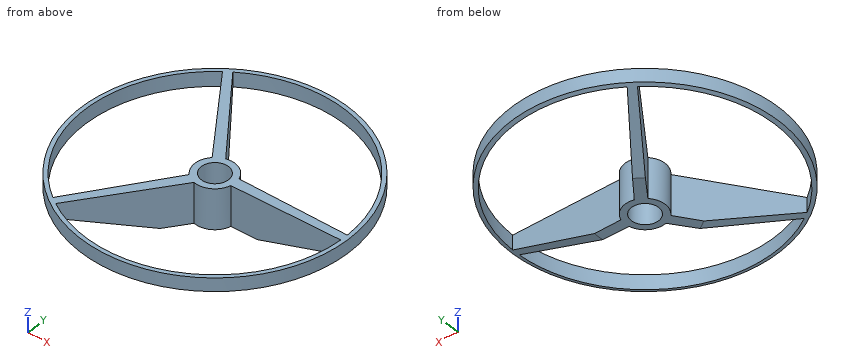
from build123d import *

# Parameters (mm, degrees)
CYLINDER_R     = 100
CYLINDER_DEPTH = 10
SKETCH_R       = 100
SKETCH_R_2     = 10.15
PAD_DEPTH      = 40


with BuildPart() as cone:
    # Cone → Cone (revolve)
    with BuildSketch(Plane(origin=(0, 0, -30), x_dir=(1, 0, 0), z_dir=(0, -1, 0))):
        Polygon((0, 0), (2, 0), (100, 30), (0, 30), align=None)
    revolve(axis=Axis((0, 0, -30), (0, 0, 1)))


with BuildPart() as fusion:
    # Cylinder → Cylinder (new body)
    with BuildSketch(Plane.XY):
        Circle(CYLINDER_R)
    extrude(amount=CYLINDER_DEPTH)

    # Fusion: union Cone
    add(cone.part)


with BuildPart() as fusion_1:
    # Fusion placement: moved
    add(fusion.part.moved(Location((0, 0, 20))))


with BuildPart() as common:
    # Sketch → Pad (new body)
    with BuildSketch(Plane.XY):
        Circle(SKETCH_R)
        Circle(SKETCH_R_2, mode=Mode.SUBTRACT)
        with BuildLine():
            ThreePointArc((96.949765, 3.121375), (44.731918, 86.070062), (-53.160067, 81.135734))
            Line((-3.811001, 14.5078), (-53.160067, 81.135734))
            ThreePointArc((14.25383, 4.672079), (7.172763, 13.173894), (-3.811001, 14.5078))
            Line((14.25383, 4.672079), (96.949765, 3.121375))
        make_face(mode=Mode.SUBTRACT)
        with BuildLine():
            Line((14.628164, -3.319158), (96.957277, -2.87862))
            ThreePointArc((-53.160067, -81.135734), (44.839635, -86.013994), (96.957277, -2.87862))
            Line((-3.811001, -14.5078), (-53.160067, -81.135734))
            ThreePointArc((-3.811001, -14.5078), (7.781336, -12.823838), (14.628164, -3.319158))
        make_face(mode=Mode.SUBTRACT)
        with BuildLine():
            Line((-10.726301, -10.485536), (-58.074672, -77.693838))
            ThreePointArc((-58.074672, 77.693838), (-97, 0), (-58.074672, -77.693838))
            Line((-10.726301, 10.485536), (-58.074672, 77.693838))
            ThreePointArc((-10.726301, 10.485536), (-15, 0), (-10.726301, -10.485536))
        make_face(mode=Mode.SUBTRACT)
    extrude(amount=PAD_DEPTH)

    # Common: intersect Fusion
    add(fusion_1.part, mode=Mode.INTERSECT)


solid = common.part
For this review, take the finished solid that the model builds, in its own axes (mm). Give positions to 0.01 mm unless a question says otherwise; leave off trailing zeros. Loops run counter-clockwise (first coordinate to the right, second up) from the corner with the lowest first, then second, coordinate; pieces in that order, holes last. Notation, with made-up numbers: M 32,-28 L 39,-28 A13 cw 39,-3 Z; hole C 61,-5 d4. An arc over 180 degrees is marked long. Answer as a JSON object with one key per item and string values. Group by question number.
Q1. Add section B-B on y = 0. Give the boundary of the cut face in (x, z).
Q2. Add section A-A on x = 0. Give the boundary of the cut face in (y, z), and give its area (3 significant figures).
Q3. For probe 1 along Y at (x, z) = (0, 18.5); probe 2 along X at (y, z) = (-71, 25.5); probe 3 along X at (y, z) = (28, 20.5), list the stretches that pass through material, from the lowest coordinate up. Write a range as [from, to].
Q4. Insertion check: P1, Ø6, axis at x = 69.5, z = 11.5, coming from the -Y side; P2, Ø5, axis at x = 56, z = 12, coming from the -Y side; P3, Ø1, axis at x = -8, z = 23.5, coming from the +Y side. Each pin has a flat end and moves straight along its axis. Give the tip position at first contact, or say it passes through.
Q5. Add section D-D on x = 85. Give the number of separate pieces and of enclosed holes in the cut face, and give its area (3 significant figures).
Q6. Add section C-C on z = 8.5. Give the boundary of the cut face in (x, y), and give its area (3 significant figures).
Checked values:
{
 "1": {"outline": "M -100,20 L -97,19.08 L -97,30 L -100,30 Z; M -15,0 L -10.15,0 L -10.15,30 L -15,30 Z; M 10.15,0 L 34.67,0 L 100,20 L 100,30 L 10.15,30 Z"},
 "2": {"outline": "M -100,20 L -97,19.08 L -97,30 L -100,30 Z; M -15,0 L -10.15,0 L -10.15,30 L -15,30 Z; M 10.15,0 L 15,0 L 15,30 L 10.15,30 Z; M 97,19.08 L 100,20 L 100,30 L 97,30 Z", "area": "354 mm²"},
 "3": {"probe 1": "[-15, -10.15], [10.15, 15]", "probe 2": "[-70.42, -66.09], [-53.36, -45.65], [66.09, 70.42]", "probe 3": "[-96, -92.87], [-23.07, -13.8], [92.87, 96]"},
 "4": {"P1": "y = -3.04", "P2": "y = -3.11", "P3": "y = 99.72"},
 "5": {"separate pieces": "3", "enclosed holes": "0", "area": "216 mm²"},
 "6": {"outline": "M -38.15,-49.42 A62.43 ccw -32.53,-53.29 L -3.81,-14.51 A15 ccw 14.63,-3.32 L 62.36,-3.06 A62.43 ccw 62.32,3.77 L 14.25,4.67 A15 ccw -3.81,14.51 L -32.53,53.29 A62.43 ccw -38.15,49.42 L -10.73,10.49 A15 ccw -10.73,-10.49 Z; hole C 0,0 d20.3", "area": "1,440 mm²"}
}
